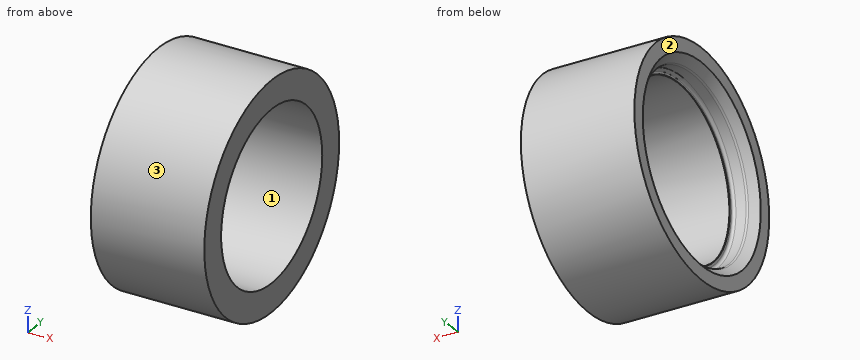
from build123d import *

# Parameters (mm, degrees)
F2_SIZE = 3
F3_R    = 1
F4_SIZE = 0.1


with BuildPart() as f1:
    # F0 (on Top) → F1 (revolve)
    with BuildSketch(Plane.XY):
        Polygon((40, 40), (0, 40), (0, 32), (8, 32), (8, 30), (40, 30), align=None)
    revolve(axis=Axis((-2.474785153, 0, 0), (1, 0, 0)))

    # F2
    f2_edges = [f1.edges().sort_by_distance(p)[0] for p in [
        (0, -32, 0),
    ]]
    chamfer(f2_edges, length=F2_SIZE)

    # F3
    f3_edges = [f1.edges().sort_by_distance(p)[0] for p in [
        (8, -32, 0),
        (3, -32, 0),
    ]]
    fillet(f3_edges, radius=F3_R)

    # F4
    f4_edges = [f1.edges().sort_by_distance(p)[0] for p in [
        (8, -30, 0),
    ]]
    chamfer(f4_edges, length=F4_SIZE)


solid = f1.part
Work out the finished part from the listing and answer in its coordinate system (mm). Face numbers are marked on the shaded views. Coordinates: 2 decimals unless noted, no trailing zeros. Write each loop counter-clockwise with the first axis right and the second up, starting at its lowest first coordinate (ties: lowest second). Pieces come first, ordered by that corner, then holes. Notation, with made-up numbers: M 53,-25.5 L 111,-25.5 A19 cw 111,-8.5 Z; hole C -13,18 d2. An arc over 180 degrees is marked long. Use one line per item in the form item = value. Start each with the question number.
1. Each of these flat-tipped pins is pushed along its axis until it touches: P1, Ø12, axis at x = 28, y = 9.5, coming from the +Z side; P2, Ø3, axis at x = 17, z = 17, coming from the -Y side; P3, Ø4, axis at x = 25.5, y = -29.5, coming from the -Z side. Where does it stop, or does it pass through?
2. The mould has two halves that part along Z. Classify the marked faces 1, 2 and 3: released by +Z, released by -Z, zero draft, split by the parting line, or undercut.
3. Straight lines are drawn through the part: probe 1 along Z at (x, y) = (21, 0); probe 2 along Z at (x, y) = (4, 0); probe 3 along Y at (x, z) = (27, -2). For each, find the intervals that lie inside material, in ascending order. Write a range as from..to.
4. The part is cut by section B-B (x = 29.5). Give the vertices of the cut face in (y, z).
5. The part is cut by section A-A (x = 4.5). Give the vertices of the cut face in (y, z).
Evaluation:
q1.P1 = 39.85
q1.P2 = -36.87
q1.P3 = -29.05
q2.face_1 = undercut
q2.face_2 = zero draft
q2.face_3 = split by the parting line
q3.probe_1 = -40..-30, 30..40
q3.probe_2 = -40..-32, 32..40
q3.probe_3 = -39.95..-29.93, 29.93..39.95
q4.outline = C 0,0 d80; hole C 0,0 d60
q5.outline = C 0,0 d80; hole C 0,0 d64
